Could you check a few things on this drawing? It's one solid part, dimensions in mm from its lowest x, y, z. Round coordinates to 2 decimals unless told otherwise and drop trailing zeros. Order: outer loops, then holes, each group sorted by start corner. A loop starts at its lowest first (then second) coordinate and runs counter-clockwise, first axis right, second up. Notation, with made-up numbers: (36, -1.5) -> (75, -1.5) arc R26 cw to (75, 23.5) -> close; hole circle Ø4 at (-23.5, -6.5). An arc over 180 degrees is marked (long way). Use a Markdown table: item, result. Add a question column.
(1) I want a section at D-D, the plane x = 9.25. Please give me the cut outline in (y, z), then the cut area to 3 significant figures.
(2) I want a section at B-B, the plane z = 1.05. Please give me the cut outline in (x, y).
(3) I want a section at C-C, the plane x = 5. Please give me the cut outline in (y, z), then the cut area to 3 significant figures.
(4) If I drill on probe 1 along Y at (x, z) = (5, 1.5); probe 2 along Y at (x, z) = (4, 2.75); probe 3 along X at (y, z) = (13.5, 2.45), over which ranges is the centre line in solid material (lowest first)?
(5) Thinking about a two-plate mould opening in X: for the marked faces 1, 2, 3 and 4, which applies, pulls with the +X half, pulls with the -X half, needs draft (parallel to the pull), parting line crosses it, or undercut?
(6) I want a section at A-A, the plane y = 12.5. Please give me the cut outline in (x, z), then the cut area to 3 significant figures.
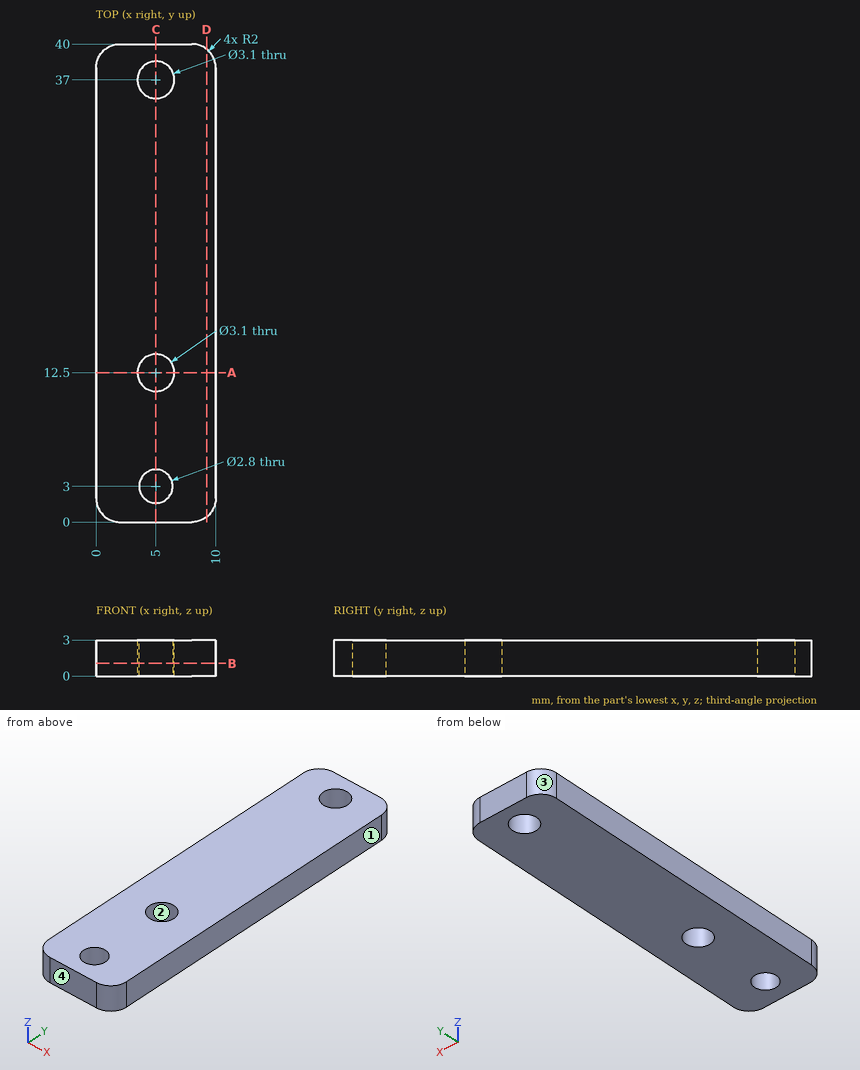
Taken from the geometry:
| question | item | result |
|---|---|---|
| 1 | outline | (0.44, 0) -> (39.56, 0) -> (39.56, 3) -> (0.44, 3) -> close |
| 1 | area | 117 mm2 |
| 2 | outline | (0, 2) arc R2 ccw to (2, 0) -> (8, 0) arc R2 ccw to (10, 2) -> (10, 38) arc R2 ccw to (8, 40) -> (2, 40) arc R2 ccw to (0, 38) -> close; hole circle Ø3.1 at (5, 12.5); hole circle Ø3.1 at (5, 37); hole circle Ø2.8 at (5, 3) |
| 3 | outline | (0, 0) -> (1.6, 0) -> (1.6, 3) -> (0, 3) -> close; (4.4, 0) -> (10.95, 0) -> (10.95, 3) -> (4.4, 3) -> close; (14.05, 0) -> (35.45, 0) -> (35.45, 3) -> (14.05, 3) -> close; (38.55, 0) -> (40, 0) -> (40, 3) -> (38.55, 3) -> close |
| 3 | area | 93.0 mm2 |
| 4 | probe 1 | y = 0 to 1.6, 4.4 to 10.95, 14.05 to 35.45, 38.55 to 40 |
| 4 | probe 2 | y = 0 to 2.02, 3.98 to 11.32, 13.68 to 35.82, 38.18 to 40 |
| 4 | probe 3 | x = 0 to 3.82, 6.18 to 10 |
| 5 | face 1 | pulls with the +X half |
| 5 | face 2 | undercut |
| 5 | face 3 | pulls with the -X half |
| 5 | face 4 | needs draft |
| 6 | outline | (0, 0) -> (3.45, 0) -> (3.45, 3) -> (0, 3) -> close; (6.55, 0) -> (10, 0) -> (10, 3) -> (6.55, 3) -> close |
| 6 | area | 20.7 mm2 |
